from build123d import *

# Parameters (mm, degrees)
SKETCH1_W           = 8
SKETCH1_H           = 15
BOSS_EXTRUDE1_DEPTH = 1
SKETCH2_R           = 1
CUT_EXTRUDE1_DEPTH  = 1


with BuildPart() as part:
    # Sketch1 → Boss-Extrude1 (new, symmetric)
    with BuildSketch(Plane.XY):
        Rectangle(SKETCH1_W, SKETCH1_H)
    extrude(amount=BOSS_EXTRUDE1_DEPTH, both=True)

    # Sketch2 → Cut-Extrude1 (cut)
    with BuildSketch(Plane(origin=(0, 0, -1), x_dir=(-1, 0, 0), z_dir=(0, 0, -1))):
        with Locations((0, 6)):
            Circle(SKETCH2_R)
        with Locations(Location((0, -6, 0), (0, 0, 180))):
            Circle(SKETCH2_R)
    extrude(amount=-CUT_EXTRUDE1_DEPTH, mode=Mode.SUBTRACT)


solid = part.part
For this review, take the finished solid that the model builds, in its own axes (mm). A direction names the side the tool comes from. Give positions to 0.01 mm unless a question says otherwise; leave off trailing zeros. Loops run counter-clockwise (first coordinate to the right, second up) from the corner with the lowest first, then second, coordinate; pieces in that order, holes last. Notation, with made-up numbers: M -35,47 L -2,47 A26 ccw -2,64 Z; hole C 81.25,-13.75 d1. An arc over 180 degrees is marked long. Answer as a JSON object with one key per item and string values. Group by question number.
Q1. Add section B-B on z = -0.75. Give the boundary of the cut face in (x, y).
Q2. Add section A-A on x = 0. Give the boundary of the cut face in (y, z), and give its area (3 significant figures).
Q3. Tool access review of faces 1 (the flat face through (4, 0, 0)), 2 (the flat face through (0, -6, 0)): name each direction out of +Z, -Z, +X, -X, +Y, -Y from which nothing blocks a thin tool from reaching the whole face with its end or side.
Q4. For probe 1 along Y at (x, z) = (0, -0.35); probe 2 along X at (y, z) = (-6, -0.15); probe 3 along Z at (x, y) = (0.5, -5.75), list the stretches that pass through material, from the lowest coordinate up. Write a range as [from, to].
Q5. Add section C-C on y = 6. Give the boundary of the cut face in (x, z).
Q6. Mouldability with a two-part tool opening along Y and no side actions: class faces 3 (the flat face through (-4, 0, 0)), 4 (the flat face through (0, -7.5, 0)), 5 (the cylindrical face through (-0.13, -6.99, -0.51)) as +Y half, -Y half, draft (parallel to the pull), parting line (faces both ways), or undercut.
Q7. Insertion check: P1, Ø1.6, axis at x = 0, y = 6.5, coming from the -Z side; P2, Ø1.2, axis at x = 0, y = 6, coming from the -Z side. Each pin has a flat end and moves straight along its axis. Give the tip position at first contact, or say it passes through.
Checked values:
{
 "1": {"outline": "M -4,-7.5 L 4,-7.5 L 4,7.5 L -4,7.5 Z; hole C 0,-6 d2; hole C 0,6 d2"},
 "2": {"outline": "M -7.5,-1 L -7,-1 L -7,0 L -5,0 L -5,-1 L 5,-1 L 5,0 L 7,0 L 7,-1 L 7.5,-1 L 7.5,1 L -7.5,1 Z", "area": "26.0 mm²"},
 "3": {"face 1": "+Z, -Z, +X, +Y, -Y", "face 2": "-Z"},
 "4": {"probe 1": "[-7.5, -7], [-5, 5], [7, 7.5]", "probe 2": "[-4, -1], [1, 4]", "probe 3": "[0, 1]"},
 "5": {"outline": "M -4,-1 L -1,-1 L -1,0 L 1,0 L 1,-1 L 4,-1 L 4,1 L -4,1 Z"},
 "6": {"face 3": "draft", "face 4": "-Y half", "face 5": "undercut"},
 "7": {"P1": "z = -1", "P2": "z = 0"}
}
